```python
from build123d import *

# Parameters (mm, degrees)
SKETCH1_R           = 20
SKETCH1_R_2         = 8.217303111
SKETCH1_R_3         = 10
BOSS_EXTRUDE1_DEPTH = 20
CUT_EXTRUDE1_DEPTH  = 20
BOSS_EXTRUDE2_REACH = 168.813


with BuildPart() as part:
    # Sketch1 → Boss-Extrude1 (new body)
    # profile 1 of 3: a face of its own
    with BuildSketch(Plane(origin=(0, 0, 0), x_dir=(1, 0, 0), z_dir=(0, 1, 0))):
        with Locations((-50, -63.493082487)):
            Circle(SKETCH1_R)
        with Locations(Location((-50, -63.493082487, 0), (0, 0, 270))):
            Circle(SKETCH1_R_2, mode=Mode.SUBTRACT)
    # profile 2 of 3: a face of its own
    with BuildSketch(Plane(origin=(0, 0, 0), x_dir=(1, 0, 0), z_dir=(0, 1, 0))):
        with Locations((50, -63.493082487)):
            Circle(SKETCH1_R)
        with Locations(Location((50, -63.493082487, 0), (0, 0, 270))):
            Circle(SKETCH1_R_3, mode=Mode.SUBTRACT)
    # profile 3 of 3: a face of its own
    with BuildSketch(Plane(origin=(0, 0, 0), x_dir=(1, 0, 0), z_dir=(0, 1, 0))):
        with BuildLine():
            Line((50, -43.493082487), (30, -43.493082487))
            Line((30, -43.493082487), (30, 96.506917513))
            Line((30, 96.506917513), (-30, 96.506917513))
            Line((-30, 96.506917513), (-30, -43.493082487))
            Line((-30, -43.493082487), (-50, -43.493082487))
            ThreePointArc((-50, -43.493082487), (-35.857864376, -49.350946863), (-30, -63.493082487))
            ThreePointArc((-30, -63.493082487), (-35.857864376, -77.635218111), (-50, -83.493082487))
            Line((-50, -83.493082487), (50, -83.493082487))
            ThreePointArc((50, -83.493082487), (30, -63.493082487), (50, -43.493082487))
        make_face()
    extrude(amount=-BOSS_EXTRUDE1_DEPTH)

    # Sketch2 → Cut-Extrude1 (cut)
    with BuildSketch(Plane(origin=(0, 0, 0), x_dir=(1, 0, 0), z_dir=(0, 1, 0))):
        with BuildLine():
            Line((-10, 96.506917513), (10, 96.506917513))
            Line((10, 96.506917513), (10, 76.506917513))
            ThreePointArc((10, 76.506917513), (0, 66.506917513), (-10, 76.506917513))
            Line((-10, 76.506917513), (-10, 96.506917513))
        make_face()
    extrude(amount=-CUT_EXTRUDE1_DEPTH, mode=Mode.SUBTRACT)

    # Sketch5 → Boss-Extrude2 (add, up to next)
    with BuildSketch(Plane(origin=(0, 41.746541244, 41.746541244), x_dir=(1, 0, 0), z_dir=(0, 0.7071067811865511, 0.707106781186544)), mode=Mode.PRIVATE) as boss_extrude2_sk1:
        with BuildLine():
            Line((-30, -8.038524809), (-30, -59.038524809))
            Line((-30, -59.038524809), (30, -59.038524809))
            Line((30, -59.038524809), (30, -8.038524809))
            ThreePointArc((30, -8.038524809), (0, -38.038524809), (-30, -8.038524809))
        make_face()
    boss_extrude2_tool1 = extrude(boss_extrude2_sk1.sketch, amount=-BOSS_EXTRUDE2_REACH, mode=Mode.PRIVATE) - part.part
    # Sketch5 → Boss-Extrude2 (add, up to next)
    with BuildSketch(Plane(origin=(0, 41.746541244, 41.746541244), x_dir=(1, 0, 0), z_dir=(0, 0.7071067811865511, 0.707106781186544)), mode=Mode.PRIVATE) as boss_extrude2_sk2:
        with BuildLine():
            ThreePointArc((30, -8.038524809), (0, 21.961475191), (-30, -8.038524809))
            Line((-30, -8.038524809), (-15, -8.038524809))
            ThreePointArc((-15, -8.038524809), (0, 6.961475191), (15, -8.038524809))
            Line((15, -8.038524809), (30, -8.038524809))
        make_face()
    boss_extrude2_tool2 = extrude(boss_extrude2_sk2.sketch, amount=-BOSS_EXTRUDE2_REACH, mode=Mode.PRIVATE) - part.part
    # Sketch5 → Boss-Extrude2 (add, up to next)
    with BuildSketch(Plane(origin=(0, 41.746541244, 41.746541244), x_dir=(1, 0, 0), z_dir=(0, 0.7071067811865511, 0.707106781186544)), mode=Mode.PRIVATE) as boss_extrude2_sk3:
        with BuildLine():
            Line((-15, -8.038524809), (-30, -8.038524809))
            ThreePointArc((-30, -8.038524809), (0, -38.038524809), (30, -8.038524809))
            Line((30, -8.038524809), (15, -8.038524809))
            ThreePointArc((15, -8.038524809), (0, -23.038524809), (-15, -8.038524809))
        make_face()
    boss_extrude2_tool3 = extrude(boss_extrude2_sk3.sketch, amount=-BOSS_EXTRUDE2_REACH, mode=Mode.PRIVATE) - part.part
    # Sketch5 → Boss-Extrude2 (add, up to next)
    with BuildSketch(Plane(origin=(0, 41.746541244, 41.746541244), x_dir=(1, 0, 0), z_dir=(0, 0.7071067811865511, 0.707106781186544)), mode=Mode.PRIVATE) as boss_extrude2_sk4:
        with BuildLine():
            ThreePointArc((30, -8.038524809), (0, 21.961475191), (-30, -8.038524809))
            Line((-30, -8.038524809), (-15, -8.038524809))
            ThreePointArc((-15, -8.038524809), (0, 6.961475191), (15, -8.038524809))
            Line((15, -8.038524809), (30, -8.038524809))
        make_face()
    boss_extrude2_tool4 = extrude(boss_extrude2_sk4.sketch, amount=-BOSS_EXTRUDE2_REACH, mode=Mode.PRIVATE) - part.part
    # Sketch5 → Boss-Extrude2 (add, up to next)
    with BuildSketch(Plane(origin=(0, 41.746541244, 41.746541244), x_dir=(1, 0, 0), z_dir=(0, 0.7071067811865511, 0.707106781186544)), mode=Mode.PRIVATE) as boss_extrude2_sk5:
        with BuildLine():
            Line((-15, -8.038524809), (-30, -8.038524809))
            ThreePointArc((-30, -8.038524809), (0, -38.038524809), (30, -8.038524809))
            Line((30, -8.038524809), (15, -8.038524809))
            ThreePointArc((15, -8.038524809), (0, -23.038524809), (-15, -8.038524809))
        make_face()
    boss_extrude2_tool5 = extrude(boss_extrude2_sk5.sketch, amount=-BOSS_EXTRUDE2_REACH, mode=Mode.PRIVATE) - part.part
    add(boss_extrude2_tool1.solids().sort_by_distance((0, 10.278536, 73.214546))[0])
    add(boss_extrude2_tool2.solids().sort_by_distance((0, 47.143389, 36.349693))[0])
    add(boss_extrude2_tool3.solids().sort_by_distance((22.5, 35.588104, 47.904978))[0])
    add(boss_extrude2_tool4.solids().sort_by_distance((0, 47.143389, 36.349693))[0])
    add(boss_extrude2_tool5.solids().sort_by_distance((22.5, 35.588104, 47.904978))[0])


solid = part.part
```
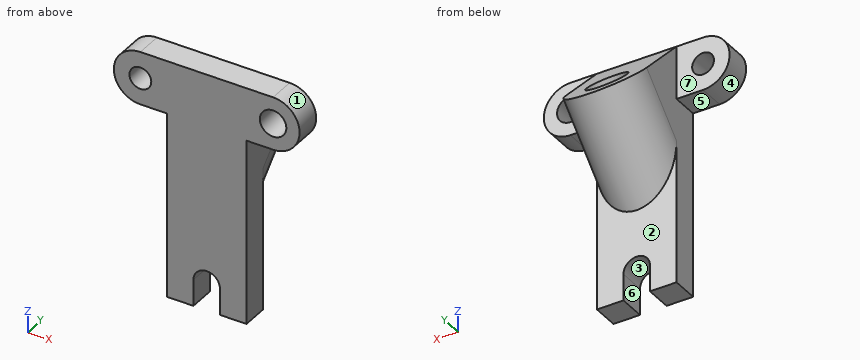
The listing builds one solid part. Answer for the finished solid, in the listing's coordinates (mm). Face numbers are marked on the shaded views. A direction names the side the tool comes from. Give positions to 0.01 mm unless a question says otherwise; leave off trailing zeros. Order: outer loops, then holes, each group sorted by start corner. A loop starts at its lowest first (then second) coordinate and runs counter-clockwise, first axis right, second up. Notation, with made-up numbers: (-27.5, 22.25) -> (-23.5, 22.25) arc R32 ccw to (-23.5, 48.25) -> close; hole circle Ø7 at (33.5, -21). An arc over 180 degrees is marked (long way). One line per item, written item: value.
1) A tool of negligible diameter and unlimited length cuts with its end or side. For the marked faces 5, 6 and 7, from which of +Z, -Z, +X, -X, +Y, -Y can it reach the whole face along a straight path? Write none if from no direction.
Reported:
face 5: -Z, -X, +Y, -Y
face 6: -Z, +Y, -Y
face 7: +Z, -Z, -X, +Y
2) Determine the mould class of the marked faces 1, 2, 3 and 4 for opening direction X: pulls with the +X half, pulls with the -X half, needs draft (parallel to the pull), parting line crosses it, or undercut.
Reported:
face 1: pulls with the +X half
face 2: needs draft
face 3: undercut
face 4: pulls with the -X half
3) Find section A-A, the plane y = -9. Determine the outline of the cut face in (x, z).
Reported:
outline: (-50, 43.49) -> (-30, 43.49) -> (-30, -96.51) -> (-10, -96.51) -> (-10, -76.51) arc R10 cw to (10, -76.51) -> (10, -96.51) -> (30, -96.51) -> (30, 43.49) -> (50, 43.49) arc R20 ccw to (50, 83.49) -> (-50, 83.49) arc R20 ccw to start; hole circle Ø16.43 at (-50, 63.49); hole circle Ø20 at (50, 63.49)
4) Find section B-B, the plane x = -46.5. Determine the outline of the cut face in (y, z), plus the area to 3 significant figures.
Reported:
outline: (-20, 43.49) -> (0, 43.49) -> (0, 56.06) -> (-20, 56.06) -> close; (-20, 70.93) -> (0, 70.93) -> (0, 83.49) -> (-20, 83.49) -> close
area: 503 mm^2
5) Flat-ended cylindrical pins translate along their axes: P1, Ø16, axis at x = 50, z = 63.49, coming from the +Y side; P2, Ø1.5, axis at y = 11.5, z = -9, coming from the +X side; P3, Ø10, axis at x = 39.5, y = -10, coming from the -Z side; P4, Ø1, axis at y = -9.5, z = 27.5, coming from the +X side. Find the tip coordinate at first contact, or state that the pin passes through.
Reported:
P1: passes through
P2: stops at x = 20.63
P3: stops at z = 43.49
P4: stops at x = 30
6) Find section D-D, the plane x = 0. Determine the outline of the cut face in (y, z).
Reported:
outline: (-20, -66.51) -> (0, -66.51) -> (0, -31.06) -> (57.28, 26.22) -> (46.67, 36.82) -> (0, -9.85) -> (0, 32.58) -> (25.46, 58.04) -> (0, 83.49) -> (-20, 83.49) -> close
7) Find section C-C, the plane z = -72. Determine the outline of the cut face in (x, y).
Reported:
outline: (-30, -20) -> (-8.93, -20) -> (-8.93, 0) -> (-30, 0) -> close; (8.93, -20) -> (30, -20) -> (30, 0) -> (8.93, 0) -> close
8) Find the intervals of material crossed by line 1 (Y direction, x = -40.5, z = 45); line 2 (X direction, y = -11.5, z = -83.5); line 3 (X direction, y = -5, z = -19), in increasing order.
Reported:
line 1: y = -20 to 0
line 2: x = -30 to -10, 10 to 30
line 3: x = -30 to 30
